```python
from build123d import *

# Parameters (mm, degrees)
SKETCH1_R           = 6
BOSS_EXTRUDE1_DEPTH = 3
SKETCH2_R           = 7
CUT_EXTRUDE1_DEPTH  = 4
SKETCH3_R           = 3.5
CUT_EXTRUDE2_DEPTH  = 4


with BuildPart() as part:
    # Sketch1 → Boss-Extrude1 (new body)
    with BuildSketch(Plane(origin=(0, 0, 0), x_dir=(1, 0, 0), z_dir=(0, 1, 0))):
        with BuildLine():
            Line((-7.092556659, 19.326923077), (87.907443341, 19.326923077))
            ThreePointArc((87.907443341, 19.326923077), (97.907443341, 9.326923077), (87.907443341, -0.673076923))
            Line((87.907443341, -0.673076923), (-7.092556659, -0.673076923))
            ThreePointArc((-7.092556659, -0.673076923), (-17.092556659, 9.326923077), (-7.092556659, 19.326923077))
        make_face()
        with Locations((-7.092556659, 9.326923077)):
            Circle(SKETCH1_R, mode=Mode.SUBTRACT)
        with Locations((87.907443341, 9.326923077)):
            Circle(SKETCH1_R, mode=Mode.SUBTRACT)
    extrude(amount=BOSS_EXTRUDE1_DEPTH)

    # Sketch2 → Cut-Extrude1 (cut, through all)
    with BuildSketch(Plane(origin=(0, 3, 0), x_dir=(1, 0, 0), z_dir=(0, 1, 0))):
        with Locations((40.407443341, 9.326923077)):
            Circle(SKETCH2_R)
    extrude(amount=-CUT_EXTRUDE1_DEPTH, mode=Mode.SUBTRACT)

    # Sketch3 → Cut-Extrude2 (cut, through all)
    with BuildSketch(Plane(origin=(0, 3, 0), x_dir=(1, 0, 0), z_dir=(0, 1, 0))):
        with Locations((17.907443341, 9.326923077)):
            Circle(SKETCH3_R)
        with Locations((62.907443341, 9.326923077)):
            Circle(SKETCH3_R)
    extrude(amount=-CUT_EXTRUDE2_DEPTH, mode=Mode.SUBTRACT)


solid = part.part
```
CAD build for the part. Positions are in the model's coordinates, mm. Round coordinates to 2 decimals unless told otherwise and drop trailing zeros. Order: outer loops, then holes, each group sorted by start corner. A loop starts at its lowest first (then second) coordinate and runs counter-clockwise, first axis right, second up. Notation, with made-up numbers: (5.5, 12.5) -> (60.5, 12.5) arc R14 cw to (60.5, 34.5) -> close; hole circle Ø2 at (-12, 49). An arc over 180 degrees is marked (long way). One line per question, with ' | ' between items.
Q1. Slice it at A-A (x = 43). Write the cut outline in (y, z).
Completed:
outline: (0, -19.33) -> (3, -19.33) -> (3, -15.83) -> (0, -15.83) -> close; (0, -2.82) -> (3, -2.82) -> (3, 0.67) -> (0, 0.67) -> close
Q2. Slice it at B-B (z = -4.5). Write the cut outline in (x, y).
Completed:
outline: (-15.85, 0) -> (-10.66, 0) -> (-10.66, 3) -> (-15.85, 3) -> close; (-3.53, 0) -> (35.34, 0) -> (35.34, 3) -> (-3.53, 3) -> close; (45.48, 0) -> (84.34, 0) -> (84.34, 3) -> (45.48, 3) -> close; (91.47, 0) -> (96.67, 0) -> (96.67, 3) -> (91.47, 3) -> close
Q3. Slice it at C-C (y = 2.3). Write the cut outline in (x, z), then the cut area to 3 significant figures.
Completed:
outline: (-7.09, -19.33) -> (87.91, -19.33) arc R10 ccw to (87.91, 0.67) -> (-7.09, 0.67) arc R10 ccw to start; hole circle Ø12 at (-7.09, -9.33); hole circle Ø7 at (17.91, -9.33); hole circle Ø14 at (40.41, -9.33); hole circle Ø7 at (62.91, -9.33); hole circle Ø12 at (87.91, -9.33) | area: 1,760 mm^2
Q4. Drop a flat-ended pin along its axis: pin 1 (7 mm diameter, centred on x = 87.91, z = -9.33, fed in from +Y) (3 decimals). Give the stop position or say it passes through.
Completed:
pin 1: passes through
Q5. Probe probe 1 along X at (y, z) = (2.3, -7.75); probe 2 along X at (y, z) = (2.05, -12.5); probe 3 along X at (y, z) = (0.95, -5). List the from-to ranges inside material, lowest first.
Completed:
probe 1: x = -16.97 to -12.88, -1.3 to 14.78, 21.03 to 33.59, 47.23 to 59.78, 66.03 to 82.12, 93.7 to 97.78 | probe 2: x = -16.58 to -12.18, -2 to 16.43, 19.38 to 34.17, 46.65 to 61.43, 64.38 to 82.82, 93 to 97.39 | probe 3: x = -16.11 to -11.25, -2.94 to 34.9, 45.91 to 83.75, 92.06 to 96.92
Q6. Slice it at D-D (x = -3.5). Write the cut outline in (y, z).
Completed:
outline: (0, -19.33) -> (3, -19.33) -> (3, -14.13) -> (0, -14.13) -> close; (0, -4.52) -> (3, -4.52) -> (3, 0.67) -> (0, 0.67) -> close
Q7. Two-plate mould, pull along Z, no slides. Class faces 1 (the cylindrical face through (-3.87, 1.48, -14.39)), 2 (the cylindrical face through (-17.09, 1.48, -9.11)), 3 (the flat face through (41, 0, -1)): released by +Z, released by -Z, zero draft, split by the parting line, or undercut.
Completed:
face 1: undercut | face 2: split by the parting line | face 3: zero draft
